```python
from build123d import *

# Parameters (mm, degrees)
SKETCH2_W                                            = 100
SKETCH2_H                                            = 210
SKETCH2_R                                            = 4
BOSS_EXTRUDE1_DEPTH                                  = 10
SKETCH3_R                                            = 2.5
MOUNT_DEPTH                                          = 11
SKETCH7_R                                            = 2.5
SUPPORT_PROFILE_MOUNT_DEPTH                          = 11
SKETCH5_R                                            = 8.5
BEARING_MOUNT_DEPTH                                  = 11
CSK_FOR_M6_SOCKET_COUNTERSUNK_HEAD_SCREW_D           = 6.6
CSK_FOR_M6_SOCKET_COUNTERSUNK_HEAD_SCREW_DEPTH       = 15
CSK_FOR_M6_SOCKET_COUNTERSUNK_HEAD_SCREW_CSINK_D     = 13.71
CSK_FOR_M6_SOCKET_COUNTERSUNK_HEAD_SCREW_CSINK_ANGLE = 90
CSK_FOR_M6_SOCKET_COUNTERSUNK_HEAD_SCREW_TIP         = 1.982840043
CSK_FOR_M5_SOCKET_COUNTERSUNK_HEAD_SCREW_D           = 5.5
CSK_FOR_M5_SOCKET_COUNTERSUNK_HEAD_SCREW_DEPTH       = 15
CSK_FOR_M5_SOCKET_COUNTERSUNK_HEAD_SCREW_CSINK_D     = 11.47
CSK_FOR_M5_SOCKET_COUNTERSUNK_HEAD_SCREW_CSINK_ANGLE = 90
CSK_FOR_M5_SOCKET_COUNTERSUNK_HEAD_SCREW_TIP         = 1.652366702


with BuildPart() as part:
    # Sketch2 → Boss-Extrude1 (new body)
    with BuildSketch(Plane(origin=(0, 0, 0), x_dir=(0, 0, -1), z_dir=(1, 0, 0))):
        with Locations((-10, 0)):
            Rectangle(SKETCH2_W, SKETCH2_H)
        with Locations((0, 88)):
            Circle(SKETCH2_R, mode=Mode.SUBTRACT)
        with Locations((0, 22)):
            Circle(SKETCH2_R, mode=Mode.SUBTRACT)
    extrude(amount=BOSS_EXTRUDE1_DEPTH)

    # Sketch3 → mount (cut, through all)
    with BuildSketch(Plane(origin=(10, 0, 0), x_dir=(0, 0, -1), z_dir=(1, 0, 0))):
        with Locations((-22.5, -70)):
            Circle(SKETCH3_R)
        with Locations((-47.5, -70)):
            Circle(SKETCH3_R)
        with Locations((-47.5, -90)):
            Circle(SKETCH3_R)
        with Locations((-22.5, -90)):
            Circle(SKETCH3_R)
        with Locations((2.5, -90)):
            Circle(SKETCH3_R)
        with Locations((27.5, -90)):
            Circle(SKETCH3_R)
        with Locations((27.5, -70)):
            Circle(SKETCH3_R)
        with Locations((2.5, -70)):
            Circle(SKETCH3_R)
    extrude(amount=-MOUNT_DEPTH, mode=Mode.SUBTRACT)

    # Sketch7 → support_profile_mount (cut, through all)
    with BuildSketch(Plane(origin=(10, 0, 0), x_dir=(0, 0, -1), z_dir=(1, 0, 0))):
        with Locations((-40, 90)):
            Circle(SKETCH7_R)
        with Locations((-40, 20)):
            Circle(SKETCH7_R)
    extrude(amount=-SUPPORT_PROFILE_MOUNT_DEPTH, mode=Mode.SUBTRACT)

    # Sketch5 → bearing_mount (cut, through all)
    with BuildSketch(Plane(origin=(10, 0, 0), x_dir=(0, 0, -1), z_dir=(1, 0, 0))):
        with Locations((0, 55)):
            Circle(SKETCH5_R)
    extrude(amount=-BEARING_MOUNT_DEPTH, mode=Mode.SUBTRACT)

    # CSK for M6 socket countersunk head screw
    with Locations(Plane.ZY):
        with Locations((40, 90), (40, 20)):
            CounterSinkHole(CSK_FOR_M6_SOCKET_COUNTERSUNK_HEAD_SCREW_D / 2, CSK_FOR_M6_SOCKET_COUNTERSUNK_HEAD_SCREW_CSINK_D / 2, depth=CSK_FOR_M6_SOCKET_COUNTERSUNK_HEAD_SCREW_DEPTH, counter_sink_angle=CSK_FOR_M6_SOCKET_COUNTERSUNK_HEAD_SCREW_CSINK_ANGLE)
            with Locations((0, 0, -(CSK_FOR_M6_SOCKET_COUNTERSUNK_HEAD_SCREW_DEPTH + CSK_FOR_M6_SOCKET_COUNTERSUNK_HEAD_SCREW_TIP / 2))):  # 118° drill point
                Cone(0, CSK_FOR_M6_SOCKET_COUNTERSUNK_HEAD_SCREW_D / 2, CSK_FOR_M6_SOCKET_COUNTERSUNK_HEAD_SCREW_TIP, mode=Mode.SUBTRACT)

    # CSK for M5 socket countersunk head screw
    with Locations(Plane.ZY):
        with Locations((-27.5, -70), (-2.5, -70), (22.5, -70), (47.5, -70), (47.5, -90), (22.5, -90), (-2.5, -90), (-27.5, -90)):
            CounterSinkHole(CSK_FOR_M5_SOCKET_COUNTERSUNK_HEAD_SCREW_D / 2, CSK_FOR_M5_SOCKET_COUNTERSUNK_HEAD_SCREW_CSINK_D / 2, depth=CSK_FOR_M5_SOCKET_COUNTERSUNK_HEAD_SCREW_DEPTH, counter_sink_angle=CSK_FOR_M5_SOCKET_COUNTERSUNK_HEAD_SCREW_CSINK_ANGLE)
            with Locations((0, 0, -(CSK_FOR_M5_SOCKET_COUNTERSUNK_HEAD_SCREW_DEPTH + CSK_FOR_M5_SOCKET_COUNTERSUNK_HEAD_SCREW_TIP / 2))):  # 118° drill point
                Cone(0, CSK_FOR_M5_SOCKET_COUNTERSUNK_HEAD_SCREW_D / 2, CSK_FOR_M5_SOCKET_COUNTERSUNK_HEAD_SCREW_TIP, mode=Mode.SUBTRACT)


solid = part.part
```
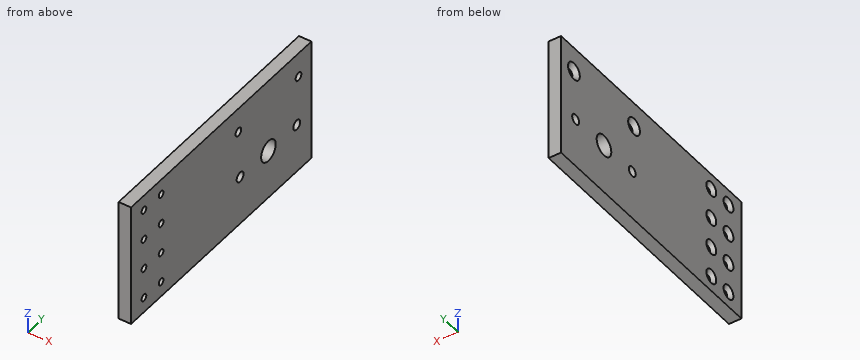
Here's how the part is built. I have some questions about the finished solid (model axes, mm). Coordinates: 2 decimals unless noted, no trailing zeros. Loops run counter-clockwise (first coordinate to the right, second up) from the corner with the lowest first, then second, coordinate; pieces in that order, holes last. Notation, with made-up numbers: M 3,85.25 L 40,85.25 A13 cw 40,109.25 Z; hole C 41.25,87 d11. An arc over 180 degrees is marked long. One line per item, written item: value.
1. Imagine slicing it at D-D (y = -70). List the corners of the cut face in (x, z) for me (3 decimals).
Geometry says:
outline: M 0,-40 L 10,-40 L 10,-30.25 L 2.985,-30.25 L 0,-33.235 Z; M 0,-21.765 L 2.985,-24.75 L 10,-24.75 L 10,-5.25 L 2.985,-5.25 L 0,-8.235 Z; M 0,3.235 L 2.985,0.25 L 10,0.25 L 10,19.75 L 2.985,19.75 L 0,16.765 Z; M 0,28.235 L 2.985,25.25 L 10,25.25 L 10,44.75 L 2.985,44.75 L 0,41.765 Z; M 0,53.235 L 2.985,50.25 L 10,50.25 L 10,60 L 0,60 Z
2. Will these pins go through, and if not, where does the flat tip stop? pin 1 Ø9 at (y, z) = (-70, 22.5) entering from -X (3 decimals); pin 2 Ø6.5 at (y, z) = (-90, 47.5) entering from -X (3 decimals).
Geometry says:
pin 1: stops at x = 1.235
pin 2: stops at x = 2.485
3. Imagine slicing it at A-A (y = 55). List the corners of the cut face in (x, z) for me, and give its area (3 significant figures).
Geometry says:
outline: M 0,-40 L 10,-40 L 10,-8.5 L 0,-8.5 Z; M 0,8.5 L 10,8.5 L 10,60 L 0,60 Z
area: 830 mm2
4. Imagine slicing it at B-B (z = 22.5). List the corners of the cut face in (x, y) for me (3 decimals).
Geometry says:
outline: M 0,-105 L 10,-105 L 10,-92.75 L 2.985,-92.75 L 0,-95.735 Z; M 0,-84.265 L 2.985,-87.25 L 10,-87.25 L 10,-72.75 L 2.985,-72.75 L 0,-75.735 Z; M 0,-64.265 L 2.985,-67.25 L 10,-67.25 L 10,105 L 0,105 Z
5. Imagine slicing it at C-C (x = 8.5). State how many separate pieces and enclosed holes the cut face has, and give its area (3 significant figures).
Geometry says:
separate pieces: 1
enclosed holes: 13
area: 20,400 mm2
6. Please list where these lines run through material, in increasing order: probe 1 along Y at (x, z) = (7, 39.5); probe 2 along Y at (x, z) = (4.5, 47.5); probe 3 along Z at (x, y) = (8, -70).
Geometry says:
probe 1: y = -105 to 16.74, 23.26 to 86.74, 93.26 to 105
probe 2: y = -105 to -92.75, -87.25 to -72.75, -67.25 to 105
probe 3: z = -40 to -30.25, -24.75 to -5.25, 0.25 to 19.75, 25.25 to 44.75, 50.25 to 60
